Input: part model. Units: mm. Frame: model coordinates. A direction names the side the tool comes from. Coordinates: 2 decimals unless noted, no trailing zeros. Loops run counter-clockwise (first coordinate to the right, second up) from the corner with the lowest first, then second, coordinate; pieces in that order, holes last.
Item 1: Reachability of faces 5 (the flat face through (-1, 45.974, -10)), 6 (the flat face through (-1, 1, 19.05)), 7 (the flat face through (30, 21, -41.275)), 8 (the flat face through (0, 0, -98.425)) from +Z, -Z, +X, -X, +Y, -Y: full face, straight path, thin tool, end or side. Return the list, or none.
Item 2: Contact query for flat-ended pins moving along their axis: P1, Ø2, axis at y = -18.5, z = -82.5, coming from the +X side; P2, Ø3, axis at y = 24.5, z = -62, coming from the +X side; P3, Ø12.5, axis at y = 2, z = -109, coming from the -X side. Output: stop coordinate, or through.
Item 3: Section B-B on x = 0. Return loops of the section in (y, z) (3 decimals).
Item 4: Section D-D on z = -51. Return loops of the section in (x, y) (3 decimals), and give its area (3 significant figures).
Item 5: Pull-direction query (Z, two-part tool) for faces 1 (the flat face through (57.306, 0.644, 30.007)), 2 (the flat face through (-4.762, 0, -111)), 3 (the flat face through (63, 1, 41.275)), 4 (the flat face through (71.13, -0.644, -36.345)); classes: released by +Z, released by -Z, zero draft, split by the parting line, or undercut.
Item 6: Ray query, line 1 along Z through (x, y) = (-24, -42) (3 decimals); line 2 along X through (y, z) = (21.5, 34); line 3 along Z through (x, y) = (24.5, -14.5) (3 decimals). Return the intervals inside material, ascending.
Item 7: Section A-A on x = 60. Return loops of the section in (y, z) (3 decimals).
```python
from build123d import *

# Parameters (mm, degrees)
BOSS_EXTRUDE1_DEPTH = 45.974
SKETCH2_R           = 34.925
BOSS_EXTRUDE2_DEPTH = 31.75
SKETCH3_R           = 19.05
BOSS_EXTRUDE3_DEPTH = 50.8
CUT_EXTRUDE1_START  = -25.4
CUT_EXTRUDE1_DEPTH  = 25.4
CHAMFER1_SIZE       = 10


with BuildPart() as part:
    # Sketch1 → Boss-Extrude1 (new, symmetric)
    with BuildSketch(Plane(origin=(0, 0, 0), x_dir=(1, 0, 0), z_dir=(0, 1, 0))):
        Polygon((-50.8, -41.275), (-63.631609733, -19.05), (63.631609733, -19.05), (50.8, -41.275), (76.2, -41.275), (76.2, 41.275), (-76.2, 41.275), (-76.2, -41.275), align=None)
    extrude(amount=BOSS_EXTRUDE1_DEPTH, both=True)

    # Sketch2 → Boss-Extrude2 (add)
    with BuildSketch(Plane(origin=(0, 0, -41.275), x_dir=(-1, 0, 0), z_dir=(0, 0, -1))):
        Circle(SKETCH2_R)
    extrude(amount=BOSS_EXTRUDE2_DEPTH)

    # Sketch3 → Boss-Extrude3 (add)
    with BuildSketch(Plane(origin=(0, 0, -73.025), x_dir=(-1, 0, 0), z_dir=(0, 0, -1))):
        Circle(SKETCH3_R)
    extrude(amount=BOSS_EXTRUDE3_DEPTH)

    # Sketch4 → Cut-Extrude1 (cut)
    with BuildSketch(Plane(origin=(0, 0, -123.825), x_dir=(-1, 0, 0), z_dir=(0, 0, -1)).offset(CUT_EXTRUDE1_START)):
        with BuildLine():
            Line((-4.7625, 18.445083186), (-4.7625, -18.445083186))
            ThreePointArc((-4.7625, -18.445083186), (0, -19.05), (4.7625, -18.445083186))
            Line((4.7625, -18.445083186), (4.7625, 18.445083186))
            ThreePointArc((4.7625, 18.445083186), (0, 19.05), (-4.7625, 18.445083186))
        make_face()
    extrude(amount=CUT_EXTRUDE1_DEPTH, mode=Mode.SUBTRACT)

    # Chamfer1
    chamfer1_edges = [part.edges().sort_by_distance(p)[0] for p in [
        (-76.2, 0, -41.275),
        (76.2, 0, -41.275),
    ]]
    chamfer(chamfer1_edges, length=CHAMFER1_SIZE)


solid = part.part
```
Results found:
1. face 5: +Z, -Z, +X, -X, +Y
1. face 6: +Y, -Y
1. face 7: -Z
1. face 8: -Z, +Y, -Y
2. P1: stops at x = 7.53
2. P2: stops at x = 26.28
2. P3: stops at x = -19.05
3. outline: (-45.974, -41.275) - (-34.925, -41.275) - (-34.925, -73.025) - (-19.05, -73.025) - (-19.05, -98.425) - (19.05, -98.425) - (19.05, -73.025) - (34.925, -73.025) - (34.925, -41.275) - (45.974, -41.275) - (45.974, 19.05) - (-45.974, 19.05) - close
4. outline: circle Ø69.85 at (0, 0)
4. area: 3,830 mm2
5. face 1: undercut
5. face 2: zero draft
5. face 3: released by +Z
5. face 4: released by -Z
6. line 1: z = -41.275 to 19.05
6. line 2: x = -76.2 to -55, 55 to 76.2
6. line 3: z = -73.025 to 19.05
7. outline: (-45.974, -41.275) - (45.974, -41.275) - (45.974, 19.05) - (-45.974, 19.05) - close; (-45.974, 25.34) - (45.974, 25.34) - (45.974, 41.275) - (-45.974, 41.275) - close
